Study the drawing (mm; zero at the part's minimum x, y, z) and answer. Coordinates: 2 decimals unless noted, no trailing zeros. Loops run counter-clockwise (first coordinate to the right, second up) from the corner with the lowest first, then second, coordinate; pieces in that order, holes last. Notation, with made-up numbers: (-22.75, 68) - (-13.75, 68) arc R22 cw to (-13.75, 87) - close; hole circle Ø1 at (60.25, 83). An arc over 180 degrees is marked (long way). One line per item, written item: value. Start each with the question number.
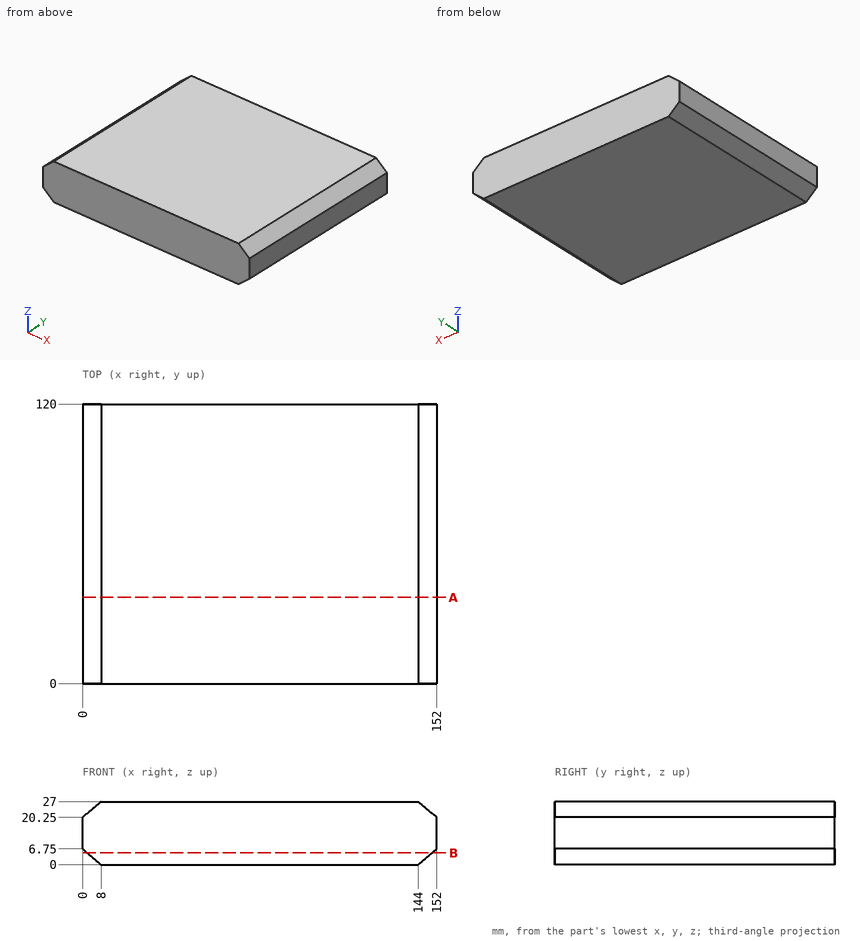
1) Section A-A, the plane y = 37 is taken. Determine the outline of the cut face in (x, z), and give its area (3 significant figures).
2) Straight lines are drawn through the part: L1, parallel to X at y = 55, z = 2.75; L2, parallel to X at y = 113, z = 20.5. For each, find the intervals that lie inside material, in ascending order.
3) Section B-B, the plane z = 5 is taken. Determine the outline of the cut face in (x, y), and give its area (3 significant figures).
4) A flat-ended cylindrical pin translates along its axis: P1, Ø1.5, axis at y = 36.5, z = 5, coming from the +X side. Find the tip coordinate at first contact, or state that the pin passes through.
Answer below:
1. outline: (0, 6.75) - (8, 0) - (144, 0) - (152, 6.75) - (152, 20.25) - (144, 27) - (8, 27) - (0, 20.25) - close
1. area: 4,000 mm2
2. L1: 4.74 to 147.26
2. L2: 0.3 to 151.7
3. outline: (2.07, 0) - (149.93, 0) - (149.93, 120) - (2.07, 120) - close
3. area: 17,700 mm2
4. P1: x = 150.81
